```python
from build123d import *

# Parameters (mm, degrees)
SALIENTE_EXTRUIR2_DEPTH  = 35
CROQUIS4_W               = 9
CROQUIS4_H               = 15
CORTAR_EXTRUIR1_DEPTH    = 70
SALIENTE_EXTRUIR3_DEPTH  = 2.1
CROQUIS8_W               = 2.1
CROQUIS8_H               = 15
SALIENTE_EXTRUIR4_DEPTH  = 7
SALIENTE_EXTRUIR5_START  = -2.1
CROQUIS9_W               = 28
CROQUIS9_H               = 15
SALIENTE_EXTRUIR5_DEPTH  = 2.1
SALIENTE_EXTRUIR6_START  = -2.1
CROQUIS10_W              = 9
CROQUIS10_H              = 15
SALIENTE_EXTRUIR6_DEPTH  = 2.1
SALIENTE_EXTRUIR7_DEPTH  = 0.9
SALIENTE_EXTRUIR8_DEPTH  = 1.2
CROQUIS16_W              = 70
CROQUIS16_H              = 39.5
CROQUIS16_W_2            = 65.8
CROQUIS16_H_2            = 15.4
CROQUIS16_H_3            = 18.7
SALIENTE_EXTRUIR10_DEPTH = 4.1


with BuildPart() as part:
    # Croquis3 → Saliente-Extruir2 (new body)
    with BuildSketch(Plane.XY):
        Polygon((-207.232131222, -11.93013618), (-207.232131222, -18.93013618), (-207.232131222, -20.93013618), (-194.032131222, -20.93013618), (-194.032131222, -11.93013618), (-196.132131222, -11.93013618), (-196.132131222, -18.93013618), (-205.132131222, -18.93013618), (-205.132131222, -11.93013618), align=None)
    extrude(amount=SALIENTE_EXTRUIR2_DEPTH)

    # Croquis4 → Cortar-Extruir1 (cut)
    with BuildSketch(Plane(origin=(0, -18.93013618, 0), x_dir=(1, 0, 0), z_dir=(0, 1, 0))):
        with Locations((-200.632131222, -7.5)):
            Rectangle(CROQUIS4_W, CROQUIS4_H)
    extrude(amount=-CORTAR_EXTRUIR1_DEPTH, mode=Mode.SUBTRACT)

    # Croquis7 → Saliente-Extruir3 (add)
    with BuildSketch(Plane.XY.offset(35)):
        Polygon((-205.132131222, -11.93013618), (-205.132131222, 3.06986382), (-207.232131222, 3.06986382), (-207.232131222, -20.93013618), (-194.032131222, -20.93013618), (-194.032131222, 3.06986382), (-196.132131222, 3.06986382), (-196.132131222, -11.93013618), align=None)
    extrude(amount=SALIENTE_EXTRUIR3_DEPTH)

    # Croquis8 → Saliente-Extruir4 (add)
    with BuildSketch(Plane(origin=(0, 0, 35), x_dir=(-1, 0, 0), z_dir=(0, 0, -1))):
        with Locations((195.082131222, -4.43013618)):
            Rectangle(CROQUIS8_W, CROQUIS8_H)
        with Locations((206.182131222, -4.43013618)):
            Rectangle(CROQUIS8_W, CROQUIS8_H)
    extrude(amount=SALIENTE_EXTRUIR4_DEPTH)

    # Croquis9 → Saliente-Extruir5 (add)
    with BuildSketch(Plane(origin=(-194.032131222, 0, 0), x_dir=(0, 0, -1), z_dir=(1, 0, 0)).offset(SALIENTE_EXTRUIR5_START)):
        with Locations((-14, -4.43013618)):
            Rectangle(CROQUIS9_W, CROQUIS9_H)
    extrude(amount=SALIENTE_EXTRUIR5_DEPTH)

    # Croquis10 → Saliente-Extruir6 (add)
    with BuildSketch(Plane.XY.offset(37.1).offset(SALIENTE_EXTRUIR6_START)):
        with Locations((-200.632131222, -4.43013618)):
            Rectangle(CROQUIS10_W, CROQUIS10_H)
    extrude(amount=SALIENTE_EXTRUIR6_DEPTH)

    # Croquis12 → Saliente-Extruir7 (add)
    with BuildSketch(Plane(origin=(-194.032131222, 0, 0), x_dir=(0, 0, -1), z_dir=(1, 0, 0))):
        Polygon((0, 3.06986382), (0, 36.06986382), (35, 36.06986382), (35, 34.26986382), (2.1, 34.26986382), (2.1, 18.86986382), (35, 18.86986382), (35, 17.06986382), (2.1, 17.06986382), (2.1, -1.63013618), (35, -1.63013618), (35, -3.43013618), (2.1, -3.43013618), (2.1, -20.93013618), (0, -20.93013618), align=None)
    extrude(amount=-SALIENTE_EXTRUIR7_DEPTH)

    # Simetría5: part across plane


with BuildPart() as part_1:
    add(part.part)
    add(part.part.mirror(Plane(origin=(0, 0, -35), x_dir=(1, 0, 0), z_dir=(0, 0, -1))))

    # Croquis13 → Saliente-Extruir8 (add)
    with BuildSketch(Plane.XZ.offset(20.93013618)):
        with BuildLine():
            Line((-194.032131222, 37.1), (-194.032131222, -2.1))
            ThreePointArc((-194.032131222, -2.1), (-174.432131222, 17.5), (-194.032131222, 37.1))
        make_face()
        with BuildLine():
            Line((-194.032131222, -67.9), (-194.032131222, -107.1))
            ThreePointArc((-194.032131222, -107.1), (-174.432131222, -87.5), (-194.032131222, -67.9))
        make_face()
    extrude(amount=-SALIENTE_EXTRUIR8_DEPTH)

    # Croquis16 → Saliente-Extruir10 (add)
    with BuildSketch(Plane(origin=(-194.032131222, 0, 0), x_dir=(0, 0, -1), z_dir=(1, 0, 0))):
        with Locations((35, 16.31986382)):
            Rectangle(CROQUIS16_W, CROQUIS16_H)
        with Locations((35, 26.56986382)):
            Rectangle(CROQUIS16_W_2, CROQUIS16_H_2, mode=Mode.SUBTRACT)
        with Locations((35, 7.71986382)):
            Rectangle(CROQUIS16_W_2, CROQUIS16_H_3, mode=Mode.SUBTRACT)
    extrude(amount=SALIENTE_EXTRUIR10_DEPTH)


solid = part_1.part
```
Design review of the part built by this model. Coordinates are the model's own, in mm. A direction names the side the tool comes from. Coordinates: 2 decimals unless noted, no trailing zeros. Order: outer loops, then holes, each group sorted by start corner. A loop starts at its lowest first (then second) coordinate and runs counter-clockwise, first axis right, second up. Notation, with made-up numbers: M 53,75.25 L 85,75.25 A31 ccw 85,105.25 Z; hole C 52,-4.5 d7. An arc over 180 degrees is marked long. Answer as a JSON object with one key per item and string values. Group by question number.
1) Wall thickness on L1, parallel to Z at x = -196, y = -12; L2, parallel to Y at x = -192, z = -65.5; L3, parallel to Z at x = -193.5, y = 3: over which ranges is each line inside the solid? List them lowest first.
2) Add section B-B, the plane z = -24. Write out the cut boundary in (x, y).
3) Add section A-A, the plane x = -200. Write out the cut boundary in (y, z).
4) Tool access review of faces 4 (the flat face through (-192, 8, -67.9)), 5 (the flat face through (-201, -8, -105)), 6 (the flat face through (-201, -9, 37.1)): name each direction out of +Z, -Z, +X, -X, +Y, -Y from which nothing blocks a thin tool from reaching the whole face with its end or side.
5) For pin 1 (1.5 mm diameter, centred on x = -193, y = 14, fed in from +Z); pin 2 (7 mm diameter, centred on y = -8, z = -88, fed in from +X); pin 3 (4 mm diameter, centred on x = -202, z = -84.5, fed in from +Y), all flat-tipped, find the tip position at first contact; note any pin that passes through.
6) Mouldability with a two-part tool opening along X and no side actions: class faces 1 (the flat face through (-192, -3.43, -35)), 2 (the flat face through (-194.932, 18, -35)), 3 (the flat face through (-201, -18.93, -95)) as pulls with the +X half, pulls with the -X half, needs draft (parallel to the pull), parting line crosses it, or undercut.
7) Add section D-D, the plane z = 17.5. Write out the cut boundary in (x, y), then the cut area to 3 significant figures.
8) Add section C-C, the plane y = 14. Write out the cut boundary in (x, z).
Computed values:
{
 "1": {"L1": "z = -107.1 to -70, 0 to 37.1", "L2": "y = -3.43 to -1.63, 17.07 to 18.87, 34.27 to 36.07", "L3": "z = -70 to -67.9, -2.1 to 0"},
 "2": {"outline": "M -194.93,-3.43 L -189.93,-3.43 L -189.93,-1.63 L -194.93,-1.63 Z; M -194.93,17.07 L -189.93,17.07 L -189.93,18.87 L -194.93,18.87 Z; M -194.93,34.27 L -189.93,34.27 L -189.93,36.07 L -194.93,36.07 Z"},
 "3": {"outline": "M -20.93,-107.1 L 3.07,-107.1 L 3.07,-105 L -18.93,-105 L -18.93,-85 L -20.93,-85 Z; M -20.93,15 L -18.93,15 L -18.93,35 L 3.07,35 L 3.07,37.1 L -20.93,37.1 Z"},
 "4": {"face 4": "+X, -X", "face 5": "+Y", "face 6": "+Z, +X, -X, +Y, -Y"},
 "5": {"pin 1": "stops at z = 0", "pin 2": "stops at x = -194.03", "pin 3": "stops at y = -18.93"},
 "6": {"face 1": "needs draft", "face 2": "pulls with the -X half", "face 3": "undercut"},
 "7": {"outline": "M -207.23,-20.93 L -174.43,-20.93 L -174.43,-19.73 L -194.03,-19.73 L -194.03,3.07 L -196.13,3.07 L -196.13,-18.93 L -205.13,-18.93 L -205.13,-11.93 L -207.23,-11.93 Z", "area": "111 mm^2"},
 "8": {"outline": "M -194.93,-70 L -189.93,-70 L -189.93,-67.9 L -194.93,-67.9 Z; M -194.93,-2.1 L -189.93,-2.1 L -189.93,0 L -194.93,0 Z"}
}
